Part model, mm, in its own coordinate system. Face numbers are marked on the shaded views. Round coordinates to 2 decimals unless told otherwise and drop trailing zeros. Order: outer loops, then holes, each group sorted by start corner. A loop starts at its lowest first (then second) coordinate and runs counter-clockwise, first axis right, second up. Notation, with made-up numbers: (34, 8) - (77, 8) arc R14 cw to (77, 32) - close; hole circle Ø10 at (53.5, 66). An arc over 180 degrees is marked (long way). Return JSON: item names as keys, results as strings. Group by question number.
Item 1: Probe probe 1 along X at (y, z) = (0.35, 0); probe 2 along X at (y, z) = (1.15, -0.75); probe 3 along Z at (x, y) = (0, 3.5). List the from-to ranges inside material, lowest first.
Item 2: Saw through at C-C on x = 1. List the corners of the cut face in (y, z).
Item 3: Saw through at A-A on z = 0. List the corners of the cut face in (x, y), and give its area (3 significant figures).
Item 4: Two-plate mould, pull along Z, no slides. Class the marked faces 1, 2 and 3: released by +Z, released by -Z, zero draft, split by the parting line, or undercut.
Item 5: Saw through at D-D on y = 2.65. State how many separate pieces and enclosed holes the cut face has, and give its area (3 significant figures).
Item 6: Drop flat-ended pins along their axis: pin 1 (1.5 mm diameter, centred on x = -9, y = 3.5, fed in from -Z); pin 2 (5 mm diameter, centred on x = 0, z = 0, fed in from -Y). Give the stop position or say it passes through.
Item 7: Saw through at B-B on z = -3.5. List the corners of the cut face in (x, y), and give its area (3 significant figures).
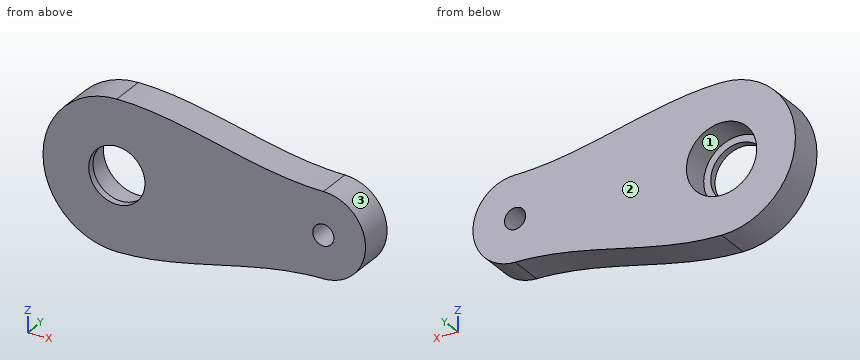
```python
from build123d import *

# Parameters (mm, degrees)
BOSS_EXTRUDE1_DEPTH = 5
SKETCH2_R           = 1.5
SKETCH2_R_2         = 5
CUT_EXTRUDE1_DEPTH  = 4
SKETCH3_R           = 4
CUT_EXTRUDE2_DEPTH  = 10
CUT_EXTRUDE3_START  = -10
SKETCH4_R           = 1.5
CUT_EXTRUDE3_DEPTH  = 10


with BuildPart() as part:
    # Sketch1 → Boss-Extrude1 (new body)
    with BuildSketch(Plane(origin=(0, 0, 0), x_dir=(1, 0, 0), z_dir=(0, 1, 0))):
        with BuildLine():
            ThreePointArc((0, -6), (6, 0), (0, 6))
            add(Edge.make_bspline(
                [(-29.37, 10.5), (-19.469048306, 10.5), (-10.126942608, 6), (0, 6)],
                knots=[0, 0, 0, 0, 1, 1, 1, 1], degree=3))
            ThreePointArc((-29.37, 10.5), (-39.87, 0), (-29.37, -10.5))
            add(Edge.make_bspline(
                [(-29.37, -10.5), (-19.469048306, -10.5), (-10.126942608, -6), (0, -6)],
                knots=[0, 0, 0, 0, 1, 1, 1, 1], degree=3))
        make_face()
    extrude(amount=BOSS_EXTRUDE1_DEPTH)

    # Sketch2 → Cut-Extrude1 (cut)
    with BuildSketch(Plane(origin=(0, 5, 0), x_dir=(1, 0, 0), z_dir=(0, 1, 0))):
        with Locations(Location((0, 0, 0), (0, 0, 270))):
            Circle(SKETCH2_R)
        with Locations(Location((-29.37, 0, 0), (0, 0, 270))):
            Circle(SKETCH2_R_2)
    extrude(amount=-CUT_EXTRUDE1_DEPTH, mode=Mode.SUBTRACT)

    # Sketch3 → Cut-Extrude2 (cut)
    with BuildSketch(Plane.XZ):
        with Locations(Location((-29.37, 0, 0), (0, 0, 270))):
            Circle(SKETCH3_R)
    extrude(amount=-CUT_EXTRUDE2_DEPTH, mode=Mode.SUBTRACT)

    # Sketch4 → Cut-Extrude3 (cut)
    with BuildSketch(Plane.XZ.offset(CUT_EXTRUDE3_START)):
        with Locations(Location((0, 0, 0), (0, 0, 90))):
            Circle(SKETCH4_R)
    extrude(amount=CUT_EXTRUDE3_DEPTH, mode=Mode.SUBTRACT)


solid = part.part
```
Filled in:
{
 "1": {"probe 1": "x = -39.87 to -33.37, -25.37 to -1.5, 1.5 to 6", "probe 2": "x = -39.84 to -34.31, -24.43 to -1.3, 1.3 to 5.95", "probe 3": "z = -6 to -1.5, 1.5 to 6"},
 "2": {"outline": "(0, -5.92) - (5, -5.92) - (5, -1.12) - (0, -1.12) - close; (0, 1.12) - (5, 1.12) - (5, 5.92) - (0, 5.92) - close"},
 "3": {"outline": "(-39.87, 0) - (-33.37, 0) - (-33.37, 1) - (-34.37, 1) - (-34.37, 5) - (-39.87, 5) - close; (-25.37, 0) - (-1.5, 0) - (-1.5, 5) - (-24.37, 5) - (-24.37, 1) - (-25.37, 1) - close; (1.5, 0) - (6, 0) - (6, 5) - (1.5, 5) - close", "area": "166 mm^2"},
 "4": {"face 1": "undercut", "face 2": "zero draft", "face 3": "split by the parting line"},
 "5": {"separate pieces": "1", "enclosed holes": "2", "area": "628 mm^2"},
 "6": {"pin 1": "stops at z = -7.13", "pin 2": "stops at y = 0"},
 "7": {"outline": "(-39.27, 0) - (-31.31, 0) - (-31.31, 1) - (-32.94, 1) - (-32.94, 5) - (-39.27, 5) - close; (-27.43, 0) - (4.87, 0) - (4.87, 5) - (-25.8, 5) - (-25.8, 1) - (-27.43, 1) - close", "area": "188 mm^2"}
}
